Read the model definition and answer for the solid it produces. Units are mm, in the model's axes. Face numbers are marked on the shaded views. Coordinates: 2 decimals unless noted, no trailing zeros. Order: outer loops, then holes, each group sorted by start corner. A loop starts at its lowest first (then second) coordinate and runs counter-clockwise, first axis right, second up.
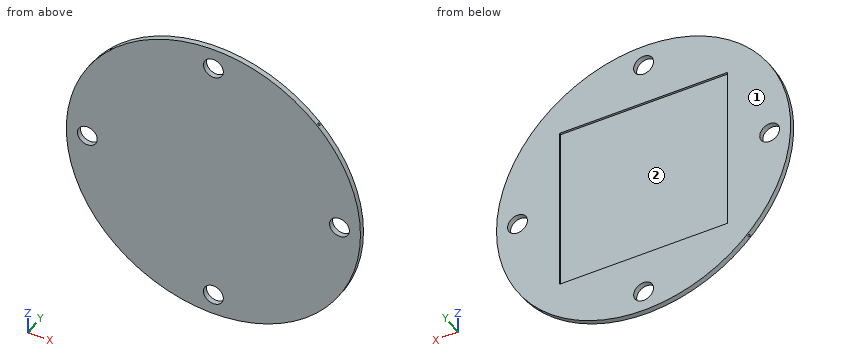
from build123d import *

# Parameters (mm, degrees)
SKETCH1_R           = 88.9
BOSS_EXTRUDE1_DEPTH = 3.175
SKETCH2_R           = 5.9944
CUT_EXTRUDE1_DEPTH  = 4.175
CIRPATTERN1_COUNT   = 4
SKETCH3_R           = 0.6985
CUT_EXTRUDE2_DEPTH  = 3.175
CIRPATTERN2_COUNT   = 4
SKETCH4_W           = 101.6
SKETCH4_H           = 101.6
CUT_EXTRUDE3_DEPTH  = 1.27


with BuildPart() as part:
    # Sketch1 → Boss-Extrude1 (new body)
    with BuildSketch(Plane(origin=(0, 0, 0), x_dir=(1, 0, 0), z_dir=(0, 1, 0))):
        Circle(SKETCH1_R)
    extrude(amount=BOSS_EXTRUDE1_DEPTH)

    # Sketch2 → Cut-Extrude1 (cut, through all)
    with BuildSketch(Plane(origin=(0, 3.175, 0), x_dir=(1, 0, 0), z_dir=(0, 1, 0))):
        with Locations((0, 76.2)):
            Circle(SKETCH2_R)
    cut_extrude1 = extrude(amount=-CUT_EXTRUDE1_DEPTH, mode=Mode.SUBTRACT)

    # CirPattern1: Cut-Extrude1 ×4 about axis
    cirpattern1_axis = Axis((0, 0, 0), (0, 1, 0))
    for i in range(1, CIRPATTERN1_COUNT):
        add(cut_extrude1.rotate(cirpattern1_axis, i * 360 / CIRPATTERN1_COUNT), mode=Mode.SUBTRACT)

    # Sketch3 → Cut-Extrude2 (cut)
    with BuildSketch(Plane(origin=(-62.861792847, 0, 62.861792847), x_dir=(0, -1, 0), z_dir=(-0.707106781, 0, 0.707106781))):
        with Locations((-1.5875, 0)):
            Circle(SKETCH3_R)
    cut_extrude2 = extrude(amount=-CUT_EXTRUDE2_DEPTH, mode=Mode.SUBTRACT)

    # CirPattern2: Cut-Extrude2 ×4 about axis
    cirpattern2_axis = Axis((0, 0, 0), (0, 1, 0))
    for i in range(1, CIRPATTERN2_COUNT):
        add(cut_extrude2.rotate(cirpattern2_axis, i * 360 / CIRPATTERN2_COUNT), mode=Mode.SUBTRACT)

    # Sketch4 → Cut-Extrude3 (cut)
    with BuildSketch(Plane(origin=(0, 3.175, 0), x_dir=(1, 0, 0), z_dir=(0, 1, 0))):
        Rectangle(SKETCH4_W, SKETCH4_H)
    extrude(amount=-CUT_EXTRUDE3_DEPTH, mode=Mode.SUBTRACT)


solid = part.part
Q1. Each of these flat-tipped pins is pushed along its axis until it touches: P1, Ø1, axis at x = -14, y = 2, coming from the -Z side; P2, Ø1, axis at y = 2.5, z = -22.5, coming from the +X side; P3, Ø7, axis at x = 76.2, z = 0, coming from the +Y side; P4, Ø1, axis at y = 1, z = -17, coming from the -X side. Where does it stop, or does it pass through?
Q2. The part is cut by section C-C, the plane x = -76.2. Determine the outline of the cut face in (y, z) (1 decimal).
Q3. The part is cut by section A-A, the plane z = 0. Determine the outline of the cut face in (x, y) (3 decimals).
Q4. The part is cut by section B-B, the plane x = 0. Determine the outline of the cut face in (y, z) (3 decimals), then the cut area to 3 significant figures.
Q5. Determine the mould class of the marked faces 1 and 2 for opening direction Z: +Z half, -Z half, draft (parallel to the pull), parting line (faces both ways), or undercut.
Q6. Straight lines are drawn through the part: L1, parallel to X at y = 2.35, z = 0; L2, parallel to Y at x = 33.5, z = 20 (3 decimals); L3, parallel to Z at x = -76.2, y = 2.3. For each, find the intervals that lie inside material, in ascending order.
Q7. The part is cut by section D-D, the plane z = 45. Determine the outline of the cut face in (x, y) (3 decimals), then the cut area to 3 significant figures.
Computed values:
1. P1: stops at z = -87.87
1. P2: stops at x = 86.13
1. P3: passes through
1. P4: stops at x = -87.36
2. outline: (0, -45.8) - (3.2, -45.8) - (3.2, -6) - (0, -6) - close; (0, 6) - (3.2, 6) - (3.2, 45.8) - (0, 45.8) - close
3. outline: (-88.9, 0) - (-82.194, 0) - (-82.194, 3.175) - (-88.9, 3.175) - close; (-70.206, 0) - (70.206, 0) - (70.206, 3.175) - (50.8, 3.175) - (50.8, 1.905) - (-50.8, 1.905) - (-50.8, 3.175) - (-70.206, 3.175) - close; (82.194, 0) - (88.9, 0) - (88.9, 3.175) - (82.194, 3.175) - close
4. outline: (0, -88.9) - (3.175, -88.9) - (3.175, -82.194) - (0, -82.194) - close; (0, -70.206) - (3.175, -70.206) - (3.175, -50.8) - (1.905, -50.8) - (1.905, 50.8) - (3.175, 50.8) - (3.175, 70.206) - (0, 70.206) - close; (0, 82.194) - (3.175, 82.194) - (3.175, 88.9) - (0, 88.9) - close
4. area: 359 mm2
5. face 1: draft
5. face 2: undercut
6. L1: x = -88.9 to -82.19, -70.21 to -50.8, 50.8 to 70.21, 82.19 to 88.9
6. L2: y = 0 to 1.905
6. L3: z = -45.79 to -5.99, 5.99 to 45.79
7. outline: (-76.669, 0) - (76.669, 0) - (76.669, 3.175) - (50.8, 3.175) - (50.8, 1.905) - (-50.8, 1.905) - (-50.8, 3.175) - (-76.669, 3.175) - close
7. area: 358 mm2
